Geometry check sheet. Reference: the model listing, model coordinates, mm. A direction names the side the tool comes from. Coordinates: 2 decimals unless noted, no trailing zeros. Loops run counter-clockwise (first coordinate to the right, second up) from the corner with the lowest first, then second, coordinate; pieces in that order, holes last.
from build123d import *

# Parameters (mm, degrees)
F1_DEPTH = 3


# Not quite as in the source:
# - a feature of the source that left no trace in its solid (it failed there, or was rolled back) is left out


with BuildPart() as f1:
    # F0 (on Top) → F1 (new body)
    with BuildSketch(Plane.XY):
        with BuildLine():
            ThreePointArc((-20.1571040975, 8.6286983024), (-18.3893371446, 7.8964652554), (-17.6571040975, 6.1286983024))
            Line((-17.6571040975, 6.1286983024), (53.465291932, 6.1286983024))
            ThreePointArc((53.465291932, 6.1286983024), (54.1975249791, 7.8964652554), (55.965291932, 8.6286983024))
            Line((55.965291932, 8.6286983024), (-20.1571040975, 8.6286983024))
        make_face()
        with BuildLine():
            Line((-18.6571040975, 6.1286983024), (-17.6571040975, 6.1286983024))
            ThreePointArc((-17.6571040975, 6.1286983024), (-18.3893371446, 7.8964652554), (-20.1571040975, 8.6286983024))
            ThreePointArc((-20.1571040975, 8.6286983024), (-22.6571040975, 6.1286983024), (-20.1571040975, 3.6286983024))
            ThreePointArc((-20.1571040975, 3.6286983024), (-18.5092794047, 4.2486254895), (-17.6786797732, 5.800959277))
            Line((-17.6786797732, 5.800959277), (-18.670049503, 5.9320548872))
            ThreePointArc((-18.670049503, 5.9320548872), (-21.6538642473, 6.2272328348), (-18.6571040975, 6.1286983024))
        make_face()
        with BuildLine():
            Line((53.465291932, 6.1286983024), (-17.6571040975, 6.1286983024))
            ThreePointArc((-17.6571040975, 6.1286983024), (-17.6625038479, 5.9644740818), (-17.6786797732, 5.800959277))
            Line((-17.6786797732, 5.800959277), (-1.2516325751, 3.6286983024))
            Line((-1.2516325751, 3.6286983024), (9.58356384, 3.6286983024))
            ThreePointArc((9.58356384, 3.6286983024), (11.4368578188, 4.4508123027), (13.2901517977, 3.6286983024))
            Line((13.2901517977, 3.6286983024), (29.319977701, 3.6286983024))
            Line((29.319977701, 3.6286983024), (53.476223752, 5.8951611635))
            ThreePointArc((53.476223752, 5.8951611635), (53.4680263825, 6.011801874), (53.465291932, 6.1286983024))
        make_face()
        with BuildLine():
            ThreePointArc((55.965291932, 8.6286983024), (54.1975249791, 7.8964652554), (53.465291932, 6.1286983024))
            Line((53.465291932, 6.1286983024), (54.465291932, 6.1286983024))
            ThreePointArc((54.465291932, 6.1286983024), (55.965291932, 7.6286983024), (57.465291932, 6.1286983024))
            ThreePointArc((57.465291932, 6.1286983024), (56.0354297891, 4.6303389727), (54.471851024, 5.9885760191))
            Line((54.471851024, 5.9885760191), (53.476223752, 5.8951611635))
            ThreePointArc((53.476223752, 5.8951611635), (54.2821167848, 4.2802066406), (55.965291932, 3.6286983024))
            ThreePointArc((55.965291932, 3.6286983024), (57.733058885, 4.3609313494), (58.465291932, 6.1286983024))
            ThreePointArc((58.465291932, 6.1286983024), (57.733058885, 7.8964652554), (55.965291932, 8.6286983024))
        make_face()
        with BuildLine():
            Line((-1.2516325751, 3.6286983024), (-17.6786797732, 5.800959277))
            ThreePointArc((-17.6786797732, 5.800959277), (-18.5092794047, 4.2486254895), (-20.1571040975, 3.6286983024))
            Line((-20.1571040975, 3.6286983024), (-1.2516325751, 3.6286983024))
        make_face()
        with BuildLine():
            ThreePointArc((55.965291932, 3.6286983024), (54.2821167848, 4.2802066406), (53.476223752, 5.8951611635))
            Line((53.476223752, 5.8951611635), (29.319977701, 3.6286983024))
            Line((29.319977701, 3.6286983024), (55.965291932, 3.6286983024))
        make_face()
        with BuildLine():
            Line((9.58356384, 3.6286983024), (-1.2516325751, 3.6286983024))
            Line((-1.2516325751, 3.6286983024), (8.9584334945, 2.2785513281))
            ThreePointArc((8.9584334945, 2.2785513281), (9.1682304635, 3.0012074295), (9.58356384, 3.6286983024))
        make_face()
        with BuildLine():
            Line((13.9259259989, 2.1843494416), (29.319977701, 3.6286983024))
            Line((29.319977701, 3.6286983024), (13.2901517977, 3.6286983024))
            ThreePointArc((13.2901517977, 3.6286983024), (13.7249931268, 2.9580048426), (13.9259259989, 2.1843494416))
        make_face()
        with BuildLine():
            ThreePointArc((9.58356384, 3.6286983024), (9.1682304635, 3.0012074295), (8.9584334945, 2.2785513281))
            Line((8.9584334945, 2.2785513281), (9.9498032243, 2.1474557179))
            ThreePointArc((9.9498032243, 2.1474557179), (11.4652982098, 3.4505426599), (12.9302987268, 2.090934586))
            Line((12.9302987268, 2.090934586), (13.9259259989, 2.1843494416))
            ThreePointArc((13.9259259989, 2.1843494416), (13.7249931268, 2.9580048426), (13.2901517977, 3.6286983024))
            Line((13.2901517977, 3.6286983024), (9.58356384, 3.6286983024))
        make_face()
        with BuildLine():
            Line((9.9498032243, 2.1474557179), (8.9584334945, 2.2785513281))
            ThreePointArc((8.9584334945, 2.2785513281), (11.2726335982, -0.5437879469), (13.9368578188, 1.9508123027))
            ThreePointArc((13.9368578188, 1.9508123027), (13.9341233684, 2.0677087311), (13.9259259989, 2.1843494416))
            Line((13.9259259989, 2.1843494416), (12.9302987268, 2.090934586))
            ThreePointArc((12.9302987268, 2.090934586), (12.9352171486, 2.0209501598), (12.9368578188, 1.9508123027))
            ThreePointArc((12.9368578188, 1.9508123027), (11.3383232865, 0.4540521529), (9.9498032243, 2.1474557179))
        make_face()
        with BuildLine():
            ThreePointArc((13.2901517977, 3.6286983024), (11.4368578188, 4.4508123027), (9.58356384, 3.6286983024))
            Line((9.58356384, 3.6286983024), (13.2901517977, 3.6286983024))
        make_face()
        with BuildLine():
            ThreePointArc((-17.6786797732, 5.800959277), (-17.6625038479, 5.9644740818), (-17.6571040975, 6.1286983024))
            Line((-17.6571040975, 6.1286983024), (-18.6571040975, 6.1286983024))
            ThreePointArc((-18.6571040975, 6.1286983024), (-18.6603439478, 6.03016377), (-18.670049503, 5.9320548872))
            Line((-18.670049503, 5.9320548872), (-17.6786797732, 5.800959277))
        make_face()
        with BuildLine():
            Line((54.465291932, 6.1286983024), (53.465291932, 6.1286983024))
            ThreePointArc((53.465291932, 6.1286983024), (53.4680263825, 6.011801874), (53.476223752, 5.8951611635))
            Line((53.476223752, 5.8951611635), (54.471851024, 5.9885760191))
            ThreePointArc((54.471851024, 5.9885760191), (54.4669326023, 6.0585604453), (54.465291932, 6.1286983024))
        make_face()
    extrude(amount=F1_DEPTH)


solid = f1.part
(1) Sectioned sample at D-D on x = 20.5. Record the cut outline in (y, z).
Findings:
outline: (2.8, 0) - (8.63, 0) - (8.63, 3) - (2.8, 3) - close
(2) Sectioned sample at A-A on z = 0.6. Record the cut outline in (x, y).
Findings:
outline: (-20.16, 3.63) - (-1.25, 3.63) - (8.96, 2.28) arc R2.5 ccw (long way) to (13.93, 2.18) - (29.32, 3.63) - (55.97, 3.63) arc R2.5 ccw to (55.97, 8.63) - (-20.16, 8.63) arc R2.5 ccw to start; hole circle Ø3 at (-20.16, 6.13); hole circle Ø3 at (11.44, 1.95); hole circle Ø3 at (55.97, 6.13)
(3) Sectioned sample at B-B on y = 1.25. Record the cut outline in (x, z), and give its area (3 significant figures).
Findings:
outline: (9.04, 0) - (10.11, 0) - (10.11, 3) - (9.04, 3) - close; (12.76, 0) - (13.84, 0) - (13.84, 3) - (12.76, 3) - close
area: 6.44 mm2
(4) Sectioned sample at C-C on x = -5. Record the cut outline in (y, z), and give its area (3 significant figures).
Findings:
outline: (3.63, 0) - (8.63, 0) - (8.63, 3) - (3.63, 3) - close
area: 15.0 mm2
(5) Gauge pin test, flat ends, axial feed: pin 1 Ø1.5 at (x, z) = (-1.5, 2) entering from -Y; pin 2 Ø4 at (x, y) = (34.5, 2) entering from +Z. Record the tip position at first contact, or that the pin passes through.
Findings:
pin 1: stops at y = 3.56
pin 2: stops at z = 3
(6) Scan lines: L1, parallel to X at y = 6, z = 2; L2, parallel to Y at x = -3, z = 2.3; L3, parallel to X at y = 0.75, z = 0.85. Record each from-to range of solid material in increasing order.
Findings:
L1: x = -22.65 to -21.65, -18.66 to 54.47, 57.46 to 58.46
L2: y = 3.63 to 8.63
L3: x = 9.24 to 10.54, 12.34 to 13.63
(7) Access from +Z, -Z, +X, -X, +Y, -Y to the whole of each face (thin tool, end or side, straight path). Record for faces 1 (the flat face through (17, 6, 0)), 2 (the flat face through (42, 3.629, 1)), 3 (the flat face through (-11, 3.629, 1)).
Findings:
face 1: -Z, +X, -X, +Y, -Y
face 2: +Z, -Z, +X, -Y
face 3: +Z, -Z, -X, -Y
